Here's how the part is built. I have some questions about the finished solid (model axes, mm). Face numbers are marked on the shaded views. A direction names the side the tool comes from. Round coordinates to 2 decimals unless told otherwise and drop trailing zeros. Order: outer loops, then holes, each group sorted by start corner. A loop starts at its lowest first (then second) coordinate and runs counter-clockwise, first axis right, second up. Notation, with made-up numbers: (84.5, 29) -> (139.5, 29) arc R19 cw to (139.5, 41) -> close; hole circle Ø10 at (21.5, -33.75). An arc over 180 degrees is marked (long way). Use a Markdown table: item, result. Add a question column.
(1) I want a section at B-B, the plane x = 15.5. Please give me the cut outline in (y, z) (3 decimals).
(2) Thinking about a two-plate mould opening in Y: for the marked faces 3, 4 and 5, which applies, pulls with the +Y half, pulls with the -Y half, needs draft (parallel to the pull), parting line crosses it, or undercut?
(3) I want a section at C-C, the plane z = 5. Please give me the cut outline in (x, y) (3 decimals), then the cut area to 3 significant figures.
(4) I want a section at A-A, the plane y = 28.5. Please give me the cut outline in (x, z) (3 decimals), then the cut area to 3 significant figures.
(5) On a 3-axis mill with a long thin cutter (end or side, diameter ignored), from which of +Z, -Z, +X, -X, +Y, -Y can I reach the whole of each face in a straight line? I mean the marked faces 1 and 2. Say none if no direction works.
(6) I'm going to push flat-ended pins straight in: P1, Ø1.9, axis at x = 12.5, z = -3.5, coming from the +Y side (3 decimals); P2, Ø5, axis at x = 11.5, y = 25.5, coming from the +Z side (3 decimals); P3, Ø3, axis at x = 8, z = -4, coming from the -Y side; P4, Ø5.5, axis at x = 18, z = 69, coming from the -Y side. Where does each tip first touch, or does it pass through?
(7) If I drill on probe 1 along Y at (x, z) = (9.75, 71) (3 decimals); probe 2 along Z at (x, y) = (22.25, 86) (3 decimals); probe 3 along X at (y, z) = (68.5, 84) (3 decimals), over which ranges is the centre line in solid material (lowest first)?
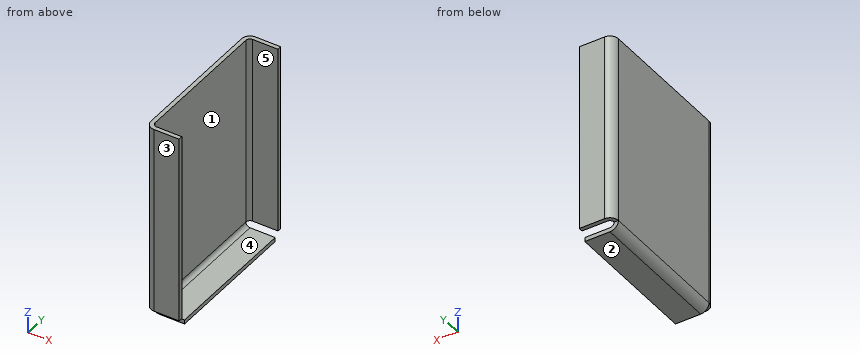
from build123d import *

# Parameters (mm, degrees)
BASE_FLANGE1_DEPTH = 142.875
EDGE_FLANGE1_DEPTH = 104.775


# Sheet-metal steps are written as plain solids
with BuildPart() as part:
    # Sketch1 → Base-Flange1 (new body)
    with BuildSketch(Plane.XY):
        with BuildLine():
            Line((25.4, 117.475), (6.35, 117.475))
            ThreePointArc((6.35, 117.475), (1.859871939, 115.615128061), (0, 111.125))
            Line((0, 111.125), (0, 6.35))
            ThreePointArc((0, 6.35), (1.859871939, 1.859871939), (6.35, 0))
            Line((6.35, 0), (25.4, 0))
            Line((25.4, 0), (25.4, 3.175))
            Line((25.4, 3.175), (6.35, 3.175))
            ThreePointArc((6.35, 3.175), (4.10493597, 4.10493597), (3.175, 6.35))
            Line((3.175, 6.35), (3.175, 111.125))
            ThreePointArc((3.175, 111.125), (4.10493597, 113.37006403), (6.35, 114.3))
            Line((6.35, 114.3), (25.4, 114.3))
            Line((25.4, 114.3), (25.4, 117.475))
        make_face()
    extrude(amount=BASE_FLANGE1_DEPTH)

    # Edge-Flange1 section (across the edge) → Edge-Flange1 (add)
    with BuildSketch(Plane(origin=(3.175, 6.35, -3.175), x_dir=(0, 0, 1), z_dir=(0, 1, 0))):
        with BuildLine():
            Line((-3.175, 3.175), (-3.175, 22.225))
            Line((-3.175, 22.225), (0, 22.225))
            Line((0, 22.225), (0, 3.175))
            ThreePointArc((0, 3.175), (0.92993597, 0.92993597), (3.175, 0))
            Line((3.175, 0), (3.175, -3.175))
            ThreePointArc((3.175, -3.175), (-1.315128061, -1.315128061), (-3.175, 3.175))
        make_face()
    extrude(amount=EDGE_FLANGE1_DEPTH)


solid = part.part
Taken from the geometry:
| question | item | result |
|---|---|---|
| 1 | outline | (0, 0) -> (3.175, 0) -> (3.175, 142.875) -> (0, 142.875) -> close; (6.35, -6.35) -> (111.125, -6.35) -> (111.125, -3.175) -> (6.35, -3.175) -> close; (114.3, 0) -> (117.475, 0) -> (117.475, 142.875) -> (114.3, 142.875) -> close |
| 2 | face 3 | pulls with the -Y half |
| 2 | face 4 | needs draft |
| 2 | face 5 | undercut |
| 3 | outline | (0, 6.35) arc R6.35 ccw to (6.35, 0) -> (25.4, 0) -> (25.4, 3.175) -> (6.35, 3.175) arc R3.175 cw to (3.175, 6.35) -> (3.175, 111.125) arc R3.175 cw to (6.35, 114.3) -> (25.4, 114.3) -> (25.4, 117.475) -> (6.35, 117.475) arc R6.35 ccw to (0, 111.125) -> close |
| 3 | area | 501 mm2 |
| 4 | outline | (0, 0) arc R6.35 ccw to (6.35, -6.35) -> (25.4, -6.35) -> (25.4, -3.175) -> (6.35, -3.175) arc R3.175 cw to (3.175, 0) -> (3.175, 142.875) -> (0, 142.875) -> close |
| 4 | area | 538 mm2 |
| 5 | face 1 | +Z, +X |
| 5 | face 2 | -Z, +X, -X, +Y, -Y |
| 6 | P1 | stops at y = 111.125 |
| 6 | P2 | stops at z = -3.175 |
| 6 | P3 | stops at y = 6.35 |
| 6 | P4 | stops at y = 0 |
| 7 | probe 1 | y = 0 to 3.175, 114.3 to 117.475 |
| 7 | probe 2 | z = -6.35 to -3.175 |
| 7 | probe 3 | x = 0 to 3.175 |
